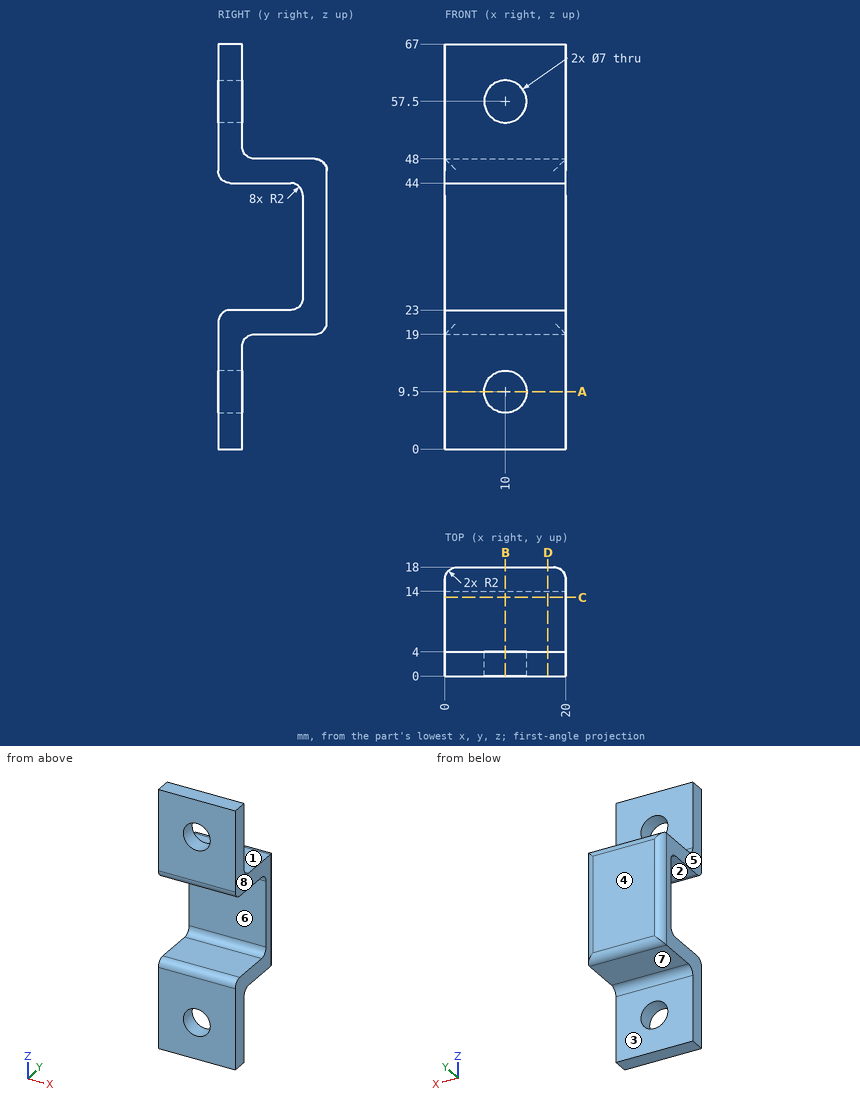
Can you work these out from the drawing? Everything is in mm from the part's minimum corner. A direction names the side the tool comes from. Round coordinates to 2 decimals unless told otherwise and drop trailing zeros. Loops run counter-clockwise (first coordinate to the right, second up) from the corner with the lowest first, then second, coordinate; pieces in that order, holes last. Notation, with made-up numbers: (-9.5, 70) -> (0.5, 70) arc R33 cw to (0.5, 98) -> close; hole circle Ø11 at (3.25, 53.25). An arc over 180 degrees is marked (long way). Put each result on its own line as item: value.
Q1. Thinking about a two-plate mould opening in Z: for the marked faces 6, 7 and 8, which applies, pulls with the +Z half, pulls with the -Z half, needs draft (parallel to the pull), parting line crosses it, or undercut?
Checks:
face 6: undercut
face 7: pulls with the -Z half
face 8: needs draft
Q2. I want a section at B-B on x = 10. Write out the boundary of the cut face in (y, z), and give its area (3 significant figures).
Checks:
outline: (0, 0) -> (4, 0) -> (4, 6) -> (0, 6) -> close; (0, 13) -> (4, 13) -> (4, 17) arc R2 cw to (6, 19) -> (16, 19) arc R2 ccw to (18, 21) -> (18, 46) arc R2 ccw to (16, 48) -> (6, 48) arc R2 cw to (4, 50) -> (4, 54) -> (0, 54) -> (0, 46) arc R2 ccw to (2, 44) -> (12, 44) arc R2 cw to (14, 42) -> (14, 25) arc R2 cw to (12, 23) -> (2, 23) arc R2 ccw to (0, 21) -> close; (0, 61) -> (4, 61) -> (4, 67) -> (0, 67) -> close
area: 324 mm2
Q3. I want a section at A-A on z = 9.5. Write out the boundary of the cut face in (x, y), and give its area (3 significant figures).
Checks:
outline: (0, 0) -> (6.5, 0) -> (6.5, 4) -> (0, 4) -> close; (13.5, 0) -> (20, 0) -> (20, 4) -> (13.5, 4) -> close
area: 52.0 mm2
Q4. For pin 1 Ø5 at (x, y) = (14.5, 10.5) entering from +Z; pin 2 Ø8 at (x, y) = (11, 11) entering from -Z; pin 3 Ø8 at (x, y) = (11, 8.5) entering from -Z, each with a flat end and sliding along its axis, tell me the tip position at first contact or that it passes through.
Checks:
pin 1: z = 48
pin 2: z = 19
pin 3: z = 18.32
Q5. Please list where these lines run through material, in increasing order: line 1 (Y direction, x = 3.5, z = 58); line 2 (Z direction, x = 15, y = 3); line 3 (X direction, y = 3, z = 9.5). Write a range as from..to.
Checks:
line 1: 0..4
line 2: 0..23, 44..67
line 3: 0..6.5, 13.5..20
Q6. I want a section at D-D on x = 17. Write out the boundary of the cut face in (y, z), and give its area (3 significant figures).
Checks:
outline: (0, 0) -> (4, 0) -> (4, 17) arc R2 cw to (6, 19) -> (16, 19) arc R2 ccw to (18, 21) -> (18, 46) arc R2 ccw to (16, 48) -> (6, 48) arc R2 cw to (4, 50) -> (4, 67) -> (0, 67) -> (0, 46) arc R2 ccw to (2, 44) -> (12, 44) arc R2 cw to (14, 42) -> (14, 25) arc R2 cw to (12, 23) -> (2, 23) arc R2 ccw to (0, 21) -> close
area: 380 mm2
Q7. I want a section at C-C on y = 13. Write out the boundary of the cut face in (x, z).
Checks:
outline: (0, 19) -> (20, 19) -> (20, 23.27) -> (0, 23.27) -> close; (0, 43.73) -> (20, 43.73) -> (20, 48) -> (0, 48) -> close
Q8. Which directions (+Z, -Z, +X, -X, +Y, -Y) give clear straight access to the entire face, cutting with the end or side of a thin tool? Please do the marked faces 1, 2, 3, 4 and 5.
Checks:
face 1: +Z, +X, -X, +Y
face 2: +X, -X, -Y
face 3: -Z, +X, -X, +Y
face 4: +Z, -Z, +X, -X, +Y
face 5: +Z, -Z, -X, +Y, -Y
